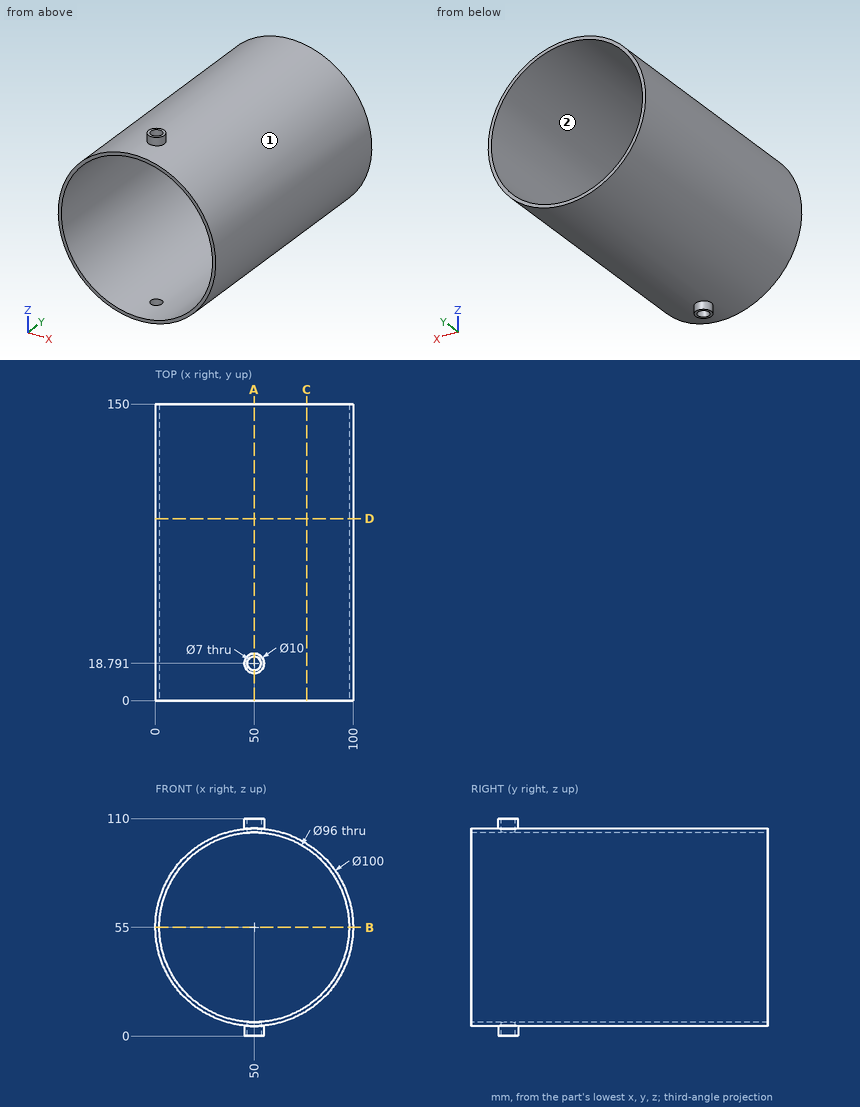
Drawing for the job (mm, zero at the part's lowest x, y, z). Round coordinates to 2 decimals unless told otherwise and drop trailing zeros. Loops run counter-clockwise (first coordinate to the right, second up) from the corner with the lowest first, then second, coordinate; pieces in that order, holes last. Notation, with made-up numbers: (30.25, 74.25) - (36.25, 74.25) arc R16 ccw to (36.25, 103.25) - close; hole circle Ø3 at (82, 50). An arc over 180 degrees is marked (long way). Write each question's results on one line, items separated by ' | '.
(1) Pin check, flat tips, straight feed: pin 1 (1 mm diameter, centred on y = 40, z = 58.5, fed in from +X); pin 2 (6 mm diameter, centred on y = 43.5, z = 17.5, fed in from -X); pin 3 (6 mm diameter, centred on y = 104.5, z = 56.5, fed in from +X). Stop position of each tip, or through.
Answer below:
pin 1: stops at x = 99.91 | pin 2: stops at x = 13.81 | pin 3: stops at x = 100
(2) Saw through at C-C, the plane x = 76.5. List the corners of the cut face in (y, z).
Answer below:
outline: (0, 12.6) - (150, 12.6) - (150, 14.98) - (0, 14.98) - close; (0, 95.02) - (150, 95.02) - (150, 97.4) - (0, 97.4) - close
(3) Saw through at A-A, the plane x = 50. List the corners of the cut face in (y, z).
Answer below:
outline: (0, 5) - (13.79, 5) - (13.79, 0) - (15.29, 0) - (15.29, 7) - (0, 7) - close; (0, 103) - (15.29, 103) - (15.29, 110) - (13.79, 110) - (13.79, 105) - (0, 105) - close; (22.29, 0) - (23.79, 0) - (23.79, 5) - (150, 5) - (150, 7) - (22.29, 7) - close; (22.29, 103) - (150, 103) - (150, 105) - (23.79, 105) - (23.79, 110) - (22.29, 110) - close
(4) Wall check: L1, parallel to X at y = 67, z = 55; L2, parallel to X at y = 139, z = 41; L3, parallel to Z at x = 56, y = 37. Give the ranges that are in metal, low to high.
Answer below:
L1: x = 0 to 2, 98 to 100 | L2: x = 2 to 4.09, 95.91 to 98 | L3: z = 5.36 to 7.38, 102.62 to 104.64
(5) Mould opens along Z. For the marked faces 1 and 2 say: released by +Z, released by -Z, zero draft, split by the parting line, or undercut.
Answer below:
face 1: split by the parting line | face 2: undercut
(6) Saw through at D-D, the plane y = 92. List the corners of the cut face in (x, z).
Answer below:
outline: circle Ø100 at (50, 55); hole circle Ø96 at (50, 55)
(7) Saw through at B-B, the plane z = 55. List the corners of the cut face in (x, y).
Answer below:
outline: (0, 0) - (2, 0) - (2, 150) - (0, 150) - close; (98, 0) - (100, 0) - (100, 150) - (98, 150) - close
